Read the model definition and answer for the solid it produces. Units are mm, in the model's axes. Face numbers are marked on the shaded views. A direction names the side the tool comes from. Coordinates: 2 decimals unless noted, no trailing zeros. Write each loop counter-clockwise with the first axis right and the second up, starting at its lowest first coordinate (ties: lowest second). Pieces come first, ordered by that corner, then holes.
(1) Which of the six approach directions +Z, -Z, +X, -X, +Y, -Y give full straight-line access (tool end or side, diameter ignored) to the marked faces 5 and 6?
(2) Given pin 1 (1 mm diameter, centred on x = -24.5, z = 149.5, fed in from -Y); pin 2 (7 mm diameter, centred on x = 5, z = 188, fed in from -Y); pin 3 (1.9 mm diameter, centred on x = -15, z = 189, fed in from +Y); pin 4 (1.5 mm diameter, centred on y = -17, z = 128.5, fed in from +X), each flat-ended and moving along its own axis, determine where each tip first touches the part or whether it passes through.
(3) Find the intervals of material crossed by probe 1 along Z at (x, y) = (-3.5, 2); probe 2 along Z at (x, y) = (-5, -45.5); probe 3 along Y at (x, z) = (32, 84.5), in increasing order.
(4) Section C-C on x = 9 is taken. Write down the section's boundary in (y, z), then the cut area to 3 significant figures.
(5) Section D-D on z = 121.5 is taken. Write down the section's boundary in (x, y).
(6) The mould has two halves that part along X. Classify the marked faces 1, 2, 3 and 4: +X half, -X half, draft (parallel to the pull), parting line (faces both ways), or undercut.
(7) Section B-B on y = 3.5 is taken. Write down the section's boundary in (x, z), then the cut area to 3 significant figures.
(8) Section A-A on x = 41 is taken. Write down the section's boundary in (y, z).
from build123d import *

# Parameters (mm, degrees)
F0_W      = 101.6
F0_H      = 101.6
F0_W_2    = 76.2
F0_H_2    = 76.2
F1_DEPTH  = 127
F2_W      = 25.4
F2_H      = 63.5
F3_DEPTH  = 25.4
F4_W      = 76.2
F4_H      = 12.7
F5_DEPTH  = 77.724
F7_DEPTH  = 25.4
F9_DEPTH  = 57.15
F10_W     = 91.44
F10_H     = 91.44
F11_DEPTH = 6.35
F12_SIZE2 = 5.08
F12_SIZE  = 5.08


with BuildPart() as f1:
    # F0 (on Top) → F1 (new body)
    with BuildSketch(Plane.XY):
        Rectangle(F0_W, F0_H)
        Rectangle(F0_W_2, F0_H_2, mode=Mode.SUBTRACT)
    extrude(amount=F1_DEPTH)

    # F2 (on face) → F3 (cut)
    with BuildSketch(Plane.XZ.offset(50.8)):
        with Locations((12.7, 31.75)):
            Rectangle(F2_W, F2_H)
    extrude(amount=-F3_DEPTH, mode=Mode.SUBTRACT)

    # F4 (on face) → F5 (join)
    with BuildSketch(Plane.XZ.offset(-38.1)):
        with Locations((0, 120.65)):
            Rectangle(F4_W, F4_H)
    extrude(amount=F5_DEPTH)

    # F6 (on face) → F7 (cut)
    with BuildSketch(Plane.XY.offset(127)):
        Polygon((-25.4, -17.603385), (-25.4, -30.303385), (25.4, -30.303385), (25.4, -17.603385), (25.4, -4.903385), (12.7, -4.903385), (12.7, -17.603385), align=None)
    extrude(amount=-F7_DEPTH, mode=Mode.SUBTRACT)

    # F8 (on face) → F9 (join)
    with BuildSketch(Plane.XY.offset(127)):
        Polygon((-23.495, -31.75), (-26.67, -28.575), (-26.67, -31.75), align=None)
        Polygon((-26.67, 28.575), (-23.495, 31.75), (-26.67, 31.75), align=None)
        Polygon((26.67, -28.575), (23.495, -31.75), (26.67, -31.75), align=None)
        Polygon((23.495, 31.75), (26.67, 28.575), (26.67, 31.75), align=None)
    extrude(amount=F9_DEPTH)

    # F10 (on face) → F11 (join)
    with BuildSketch(Plane.XY.offset(184.15)):
        Rectangle(F10_W, F10_H)
    extrude(amount=F11_DEPTH)

    # F12
    f12_edges = [f1.edges().sort_by_distance(p)[0] for p in [
        (50.8, -50.8, 63.5),
        (-50.8, -50.8, 63.5),
        (50.8, 50.8, 63.5),
        (-50.8, 50.8, 63.5),
    ]]
    chamfer(f12_edges, length=F12_SIZE, length2=F12_SIZE2)


solid = f1.part
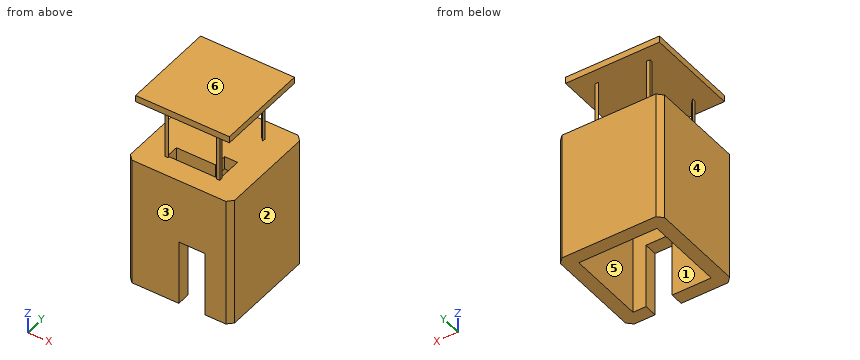
Response:
1. face 5: -Z
1. face 6: +Z, +X, -X, +Y, -Y
2. pin 1: stops at y = -31.75
2. pin 2: stops at y = -45.72
2. pin 3: stops at y = 45.72
2. pin 4: passes through
3. probe 1: z = 114.3 to 127, 184.15 to 190.5
3. probe 2: z = 0 to 127, 184.15 to 190.5
3. probe 3: y = -50.8 to -38.1, 38.1 to 50.8
4. outline: (-50.8, 63.5) - (-38.1, 63.5) - (-38.1, 114.3) - (-30.3, 114.3) - (-30.3, 127) - (-50.8, 127) - close; (-45.72, 184.15) - (45.72, 184.15) - (45.72, 190.5) - (-45.72, 190.5) - close; (-17.6, 114.3) - (38.1, 114.3) - (38.1, 0) - (50.8, 0) - (50.8, 127) - (-17.6, 127) - close
4. area: 3,810 mm2
5. outline: (-50.8, -45.72) - (-45.72, -50.8) - (45.72, -50.8) - (50.8, -45.72) - (50.8, 45.72) - (45.72, 50.8) - (-45.72, 50.8) - (-50.8, 45.72) - close; hole (-25.4, -30.3) - (25.4, -30.3) - (25.4, -4.9) - (12.7, -4.9) - (12.7, -17.6) - (-25.4, -17.6) - close
6. face 1: undercut
6. face 2: +X half
6. face 3: draft
6. face 4: -X half
7. outline: (-50.8, 0) - (-38.1, 0) - (-38.1, 114.3) - (38.1, 114.3) - (38.1, 0) - (50.8, 0) - (50.8, 127) - (-50.8, 127) - close; (-45.72, 184.15) - (45.72, 184.15) - (45.72, 190.5) - (-45.72, 190.5) - close
7. area: 4,770 mm2
8. outline: (-50.8, 0) - (50.8, 0) - (50.8, 127) - (-50.8, 127) - close; (-45.72, 184.15) - (45.72, 184.15) - (45.72, 190.5) - (-45.72, 190.5) - close
